The listing builds one solid part. Answer for the finished solid, in the listing's coordinates (mm). Face numbers are marked on the shaded views. A direction names the side the tool comes from. Round coordinates to 2 decimals unless told otherwise and drop trailing zeros. Order: outer loops, then holes, each group sorted by start corner. A loop starts at its lowest first (then second) coordinate and runs counter-clockwise, first axis right, second up. Notation, with made-up numbers: M 0,12 L 59,12 A31 cw 59,41 Z; hole C 83,-24 d3. An arc over 180 degrees is marked long. Put each result on its own line as item: value. Start each with the question number.
1. Consider line 1 (Y direction, x = 6, z = 1.5); line 2 (X direction, y = 3.5, z = 5.25); line 3 (Z direction, x = 2.5, y = -8.5). Determine where each line is inside the solid, lowest interval first.
2. The mould has two halves that part along Y. Classify the marked faces 1, 2 and 3: +Y half, -Y half, draft (parallel to the pull), parting line (faces both ways), or undercut.
3. The part is cut by section A-A (y = 2.25). Give the vertices of the cut face in (x, z), then the cut area to 3 significant figures.
4. Each of these flat-tipped pins is pushed along its axis until it touches: pin 1 Ø6 at (x, y) = (-1, -9.5) entering from -Z; pin 2 Ø1.5 at (y, z) = (-9.5, -2) entering from -X; pin 3 Ø5 at (x, y) = (-5.5, -7) entering from -Z. Where does it stop, or does it pass through?
5. Which of the six approach directions +Z, -Z, +X, -X, +Y, -Y give full straight-line access (tool end or side, diameter ignored) to the marked faces 4 and 5?
6. The part is cut by section B-B (y = -5.5). Give the vertices of the cut face in (x, z).
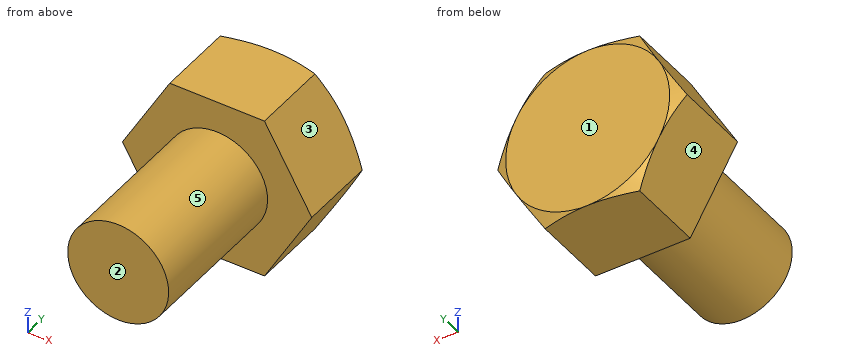
from build123d import *

# Parameters (mm, degrees)
BOSS_EXTRUDE1_DEPTH = 6.7
SKETCH2_R           = 4
BOSS_EXTRUDE2_DEPTH = 12
SKETCH3_OUTSIDE_W   = 57.108
SKETCH3_OUTSIDE_H   = 55.096
SKETCH3_OUTSIDE_R   = 6.5
CUT_EXTRUDE3_DEPTH  = 10
CUT_EXTRUDE3_DRAFT  = -60


with BuildPart() as part:
    # Sketch1 → Boss-Extrude1 (new body)
    with BuildSketch(Plane(origin=(0, 0, 0), x_dir=(1, 0, 0), z_dir=(0, 1, 0))):
        Polygon((7.505553499, 0), (3.75277675, 6.5), (-3.75277675, 6.5), (-7.505553499, 0), (-3.75277675, -6.5), (3.75277675, -6.5), align=None)
    extrude(amount=BOSS_EXTRUDE1_DEPTH)

    # Sketch2 → Boss-Extrude2 (add)
    with BuildSketch(Plane.XZ):
        with Locations(Location((0, 0, 0), (0, 0, 270))):
            Circle(SKETCH2_R)
    extrude(amount=BOSS_EXTRUDE2_DEPTH)


with BuildPart() as cut_extrude3_tool:
    # Sketch3 outside → Cut-Extrude3 (with draft: the straight prism first)
    with BuildSketch(Plane(origin=(0, 6.7, 0), x_dir=(1, 0, 0), z_dir=(0, 1, 0))):
        Rectangle(SKETCH3_OUTSIDE_W, SKETCH3_OUTSIDE_H)
        Circle(SKETCH3_OUTSIDE_R, mode=Mode.SUBTRACT)
    extrude(amount=-CUT_EXTRUDE3_DEPTH)
    # Cut-Extrude3: the draft: its side faces are tilted about the plane it starts from
    cut_extrude3_sides = [cut_extrude3_tool.faces().sort_by_distance(p)[0] for p in [
        (0, 1.7, 27.548),
        (28.554, 1.7, 0),
        (0, 1.7, -27.548),
        (-28.554, 1.7, 0),
        (-6.5, 1.7, 0),
    ]]
    draft(cut_extrude3_sides, Plane(origin=(0, 6.7, 0), x_dir=(1, 0, 0), z_dir=(0, 1, 0)), CUT_EXTRUDE3_DRAFT)


with BuildPart() as part_1:
    add(part.part)

    # Cut-Extrude3: cut by cut_extrude3_tool
    add(cut_extrude3_tool.part, mode=Mode.SUBTRACT)


solid = part_1.part
Resolved:
1. line 1: 0 to 6.7
1. line 2: -4.47 to 4.47
1. line 3: -3.12 to 3.12
2. face 1: +Y half
2. face 2: -Y half
2. face 3: draft
3. outline: M -7.51,0 L -3.75,-6.5 L 3.75,-6.5 L 7.51,0 L 3.75,6.5 L -3.75,6.5 Z
3. area: 146 mm2
4. pin 1: z = -4
4. pin 2: x = -3.8
4. pin 3: z = -2.65
5. face 4: -Z, -X, +Y, -Y
5. face 5: -Y
6. outline: C 0,0 d8
